For this review, take the finished solid that the model builds, in its own axes (mm). A direction names the side the tool comes from. Give positions to 0.01 mm unless a question says otherwise; leave off trailing zeros. Loops run counter-clockwise (first coordinate to the right, second up) from the corner with the lowest first, then second, coordinate; pieces in that order, holes last.
```python
from build123d import *

# Parameters (mm, degrees)
SKETCH001_W      = 29
SKETCH001_H      = 38
PAD_DEPTH        = 2
SKETCH_W         = 7
SKETCH_H         = 38
PAD001_DEPTH     = 14
HOLE_D           = 2.2
HOLE_DEPTH       = 25
HOLE_CSINK_D     = 3.5
HOLE_CSINK_ANGLE = 90


with BuildPart() as part:
    # Sketch001 → Pad (new body)
    with BuildSketch(Plane.XY):
        Rectangle(SKETCH001_W, SKETCH001_H)
    extrude(amount=-PAD_DEPTH)

    # Sketch → Pad001 (join)
    with BuildSketch(Plane.XY):
        with Locations((11, 0)):
            Rectangle(SKETCH_W, SKETCH_H)
        with Locations((-11, 0)):
            Rectangle(SKETCH_W, SKETCH_H)
    extrude(amount=PAD001_DEPTH)

    # Hole
    with Locations(Plane.XY):
        with Locations((0, 13.25), (0, -13.25)):
            CounterSinkHole(HOLE_D / 2, HOLE_CSINK_D / 2, depth=HOLE_DEPTH, counter_sink_angle=HOLE_CSINK_ANGLE)


solid = part.part
```
Item 1: Take a section at A-A on x = 0. Give the boundary of the cut face in (y, z), and give its area (3 significant figures).
Answer:
outline: (-19, -2) - (-14.35, -2) - (-14.35, -0.65) - (-15, 0) - (-19, 0) - close; (-12.15, -2) - (12.15, -2) - (12.15, -0.65) - (11.5, 0) - (-11.5, 0) - (-12.15, -0.65) - close; (14.35, -2) - (19, -2) - (19, 0) - (15, 0) - (14.35, -0.65) - close
area: 66.4 mm2
Item 2: For L1, parallel to Y at x = 0, z = -0.95; L2, parallel to X at y = 13.25, z = -1.5; L3, parallel to X at y = 8, z = 0.25, list the stretches that pass through material, from the lowest coordinate up.
Answer:
L1: y = -19 to -14.35, -12.15 to 12.15, 14.35 to 19
L2: x = -14.5 to -1.1, 1.1 to 14.5
L3: x = -14.5 to -7.5, 7.5 to 14.5
Item 3: Take a section at D-D on y = -0.5. Give the boundary of the cut face in (x, z).
Answer:
outline: (-14.5, -2) - (14.5, -2) - (14.5, 14) - (7.5, 14) - (7.5, 0) - (-7.5, 0) - (-7.5, 14) - (-14.5, 14) - close
Item 4: Tool access review of faces 1 (the flat face through (-14.5, 0, 6)), 2 (the flat face through (-7.5, 0, 7)): name each direction out of +Z, -Z, +X, -X, +Y, -Y from which nothing blocks a thin tool from reaching the whole face with its end or side.
Answer:
face 1: +Z, -Z, -X, +Y, -Y
face 2: +Z, +Y, -Y
Item 5: Take a section at B-B on z = 6.5. Give the boundary of the cut face in (x, y), and give its area (3 significant figures).
Answer:
outline: (-14.5, -19) - (-7.5, -19) - (-7.5, 19) - (-14.5, 19) - close; (7.5, -19) - (14.5, -19) - (14.5, 19) - (7.5, 19) - close
area: 532 mm2
Item 6: Clearance check with flat-ended pins moving along their axes: pin 1 Ø2.5 at (x, y) = (0, 13.25) entering from +Z; pin 2 Ø4.5 at (x, y) = (1, -2.5) entering from +Z; pin 3 Ø2.5 at (x, y) = (0, -13.25) entering from -Z. State where each tip first meets the part, or that it passes through.
Answer:
pin 1: stops at z = -0.5
pin 2: stops at z = 0
pin 3: stops at z = -2
Item 7: The part is to be moulded in two halves that separate along X. For faces 3 (the flat face through (0, -19, -1)), 4 (the flat face through (0, 0, 0)), 5 (the cylindrical face through (0.238, 12.176, -1.334)), 6 (the flat face through (14.5, 0, 6)), say which applies: released by +X, released by -X, zero draft, split by the parting line, or undercut.
Answer:
face 3: zero draft
face 4: undercut
face 5: undercut
face 6: released by +X
Item 8: Take a section at C-C on y = -13.25. Give the boundary of the cut face in (x, z).
Answer:
outline: (-14.5, -2) - (-1.1, -2) - (-1.1, -0.65) - (-1.75, 0) - (-7.5, 0) - (-7.5, 14) - (-14.5, 14) - close; (1.1, -2) - (14.5, -2) - (14.5, 14) - (7.5, 14) - (7.5, 0) - (1.75, 0) - (1.1, -0.65) - close
